Here's how the part is built. I have some questions about the finished solid (model axes, mm). Face numbers are marked on the shaded views. A direction names the side the tool comes from. Round coordinates to 2 decimals unless told otherwise and drop trailing zeros. Write each loop counter-clockwise with the first axis right and the second up, starting at its lowest first coordinate (ties: lowest second). Pieces come first, ordered by that corner, then holes. Notation, with made-up numbers: (32.5, -5.75) - (36.5, -5.75) arc R29 cw to (36.5, 28.25) - close; hole circle Ø2 at (50, 75.5). An arc over 180 degrees is marked (long way). One line per question, with ' | ' between items. Start each with the question number.
(1) For the marked faces 1 and 2, which set-ups out of +Z, -Z, +X, -X, +Y, -Y let a thin tool reach every point of the face, with its end or its side?
(2) Imagine slicing it at B-B (z = 2.25). Write out the boundary of the cut face in (x, y).
(3) Imagine slicing it at C-C (y = -49). Write out the boundary of the cut face in (x, z), plus the area to 3 significant figures.
(4) Thinking about a two-plate mould opening in Y: for the marked faces 3, 4, 5 and 6, which applies, pulls with the +Y half, pulls with the -Y half, needs draft (parallel to the pull), parting line crosses it, or undercut?
(5) Imagine slicing it at D-D (x = 23.5). Write out the boundary of the cut face in (y, z), plus the area to 3 significant figures.
(6) Imagine slicing it at A-A (x = -6). Write out the boundary of the cut face in (y, z).
(7) If I drill on L1, parallel to X at y = 7, z = 1.5; L2, parallel to Y at x = -22, z = 7.5; L3, parallel to Y at x = 0, z = -0.75, over which ranges is the centre line in solid material (lowest first)?
(8) Will these pins go through, and if not, where does the flat tip stop? pin 1 (10 mm diameter, centred on x = -10.5, y = -1, fed in from +Z); pin 2 (2.5 mm diameter, centred on x = -5, y = -50.5, fed in from -Z).
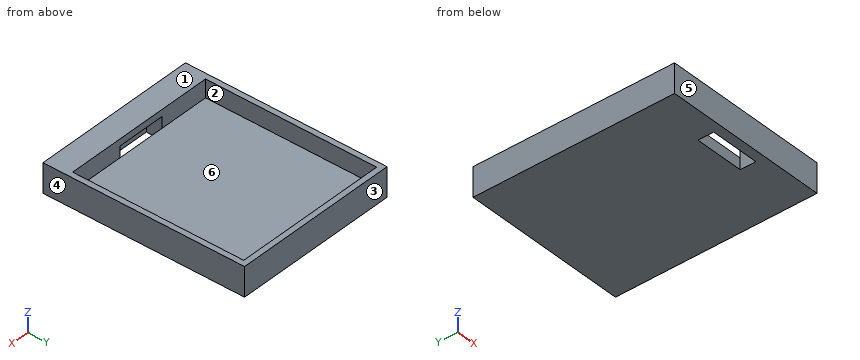
from build123d import *

# Parameters (mm, degrees)
SKETCH2_W           = 74.2
SKETCH2_H           = 90
SKETCH2_W_2         = 69.2
SKETCH2_H_2         = 76.4
BOSS_EXTRUDE1_DEPTH = 8
SKETCH3_W           = 74.2
SKETCH3_H           = 90
BOSS_EXTRUDE2_DEPTH = 5
SKETCH5_W           = 22
SKETCH5_H           = 5
CUT_EXTRUDE1_DEPTH  = 8
SKETCH9_W           = 22
SKETCH9_H           = 7
CUT_EXTRUDE2_DEPTH  = 69.755085919


with BuildPart() as part:
    # Sketch2 → Boss-Extrude1 (new body)
    with BuildSketch(Plane.XY):
        with Locations((0.944957983, -11.708403361)):
            Rectangle(SKETCH2_W, SKETCH2_H)
        with Locations((0.944957983, -7.408403361)):
            Rectangle(SKETCH2_W_2, SKETCH2_H_2, mode=Mode.SUBTRACT)
    extrude(amount=BOSS_EXTRUDE1_DEPTH)

    # Sketch3 → Boss-Extrude2 (add)
    with BuildSketch(Plane(origin=(0, 0, 0), x_dir=(-1, 0, 0), z_dir=(0, 0, -1))):
        with Locations((-0.944957983, -11.708403361)):
            Rectangle(SKETCH3_W, SKETCH3_H)
    extrude(amount=BOSS_EXTRUDE2_DEPTH)

    # Sketch5 → Cut-Extrude1 (cut)
    with BuildSketch(Plane(origin=(0, -45.608403361, 0), x_dir=(1, 0, 0), z_dir=(0, 1, 0))):
        with Locations((0, -2.5)):
            Rectangle(SKETCH5_W, SKETCH5_H)
    extrude(amount=-CUT_EXTRUDE1_DEPTH, mode=Mode.SUBTRACT)

    # Sketch9 → Cut-Extrude2 (cut, through all)
    with BuildSketch(Plane.XY):
        with Locations((0, -49.108403361)):
            Rectangle(SKETCH9_W, SKETCH9_H)
    extrude(amount=-CUT_EXTRUDE2_DEPTH, mode=Mode.SUBTRACT)


solid = part.part
Check sheet entries:
1) face 1: +Z, +X, -X, +Y, -Y | face 2: +Z
2) outline: (-36.16, -56.71) - (38.04, -56.71) - (38.04, 33.29) - (-36.16, 33.29) - close; hole (-33.66, -45.61) - (-11, -45.61) - (-11, -53.61) - (11, -53.61) - (11, -45.61) - (35.54, -45.61) - (35.54, 30.79) - (-33.66, 30.79) - close
3) outline: (-36.16, -5) - (-11, -5) - (-11, 5) - (11, 5) - (11, -5) - (38.04, -5) - (38.04, 8) - (-36.16, 8) - close | area: 745 mm^2
4) face 3: pulls with the +Y half | face 4: needs draft | face 5: pulls with the -Y half | face 6: undercut
5) outline: (-56.71, -5) - (33.29, -5) - (33.29, 8) - (30.79, 8) - (30.79, 0) - (-45.61, 0) - (-45.61, 8) - (-56.71, 8) - close | area: 559 mm^2
6) outline: (-56.71, -5) - (-52.61, -5) - (-52.61, 0) - (-53.61, 0) - (-53.61, 5) - (-45.61, 5) - (-45.61, 8) - (-56.71, 8) - close; (-45.61, -5) - (33.29, -5) - (33.29, 8) - (30.79, 8) - (30.79, 0) - (-45.61, 0) - close
7) L1: -36.16 to -33.66, 35.54 to 38.04 | L2: -56.71 to -45.61, 30.79 to 33.29 | L3: -56.71 to -52.61, -45.61 to 33.29
8) pin 1: z = 0 | pin 2: z = 5
